Source: CAD feature listing. Evaluate the final solid. Frame: model axes, mm. A direction names the side the tool comes from. Round coordinates to 2 decimals unless told otherwise and drop trailing zeros. Order: outer loops, then holes, each group sorted by start corner. A loop starts at its lowest first (then second) coordinate and runs counter-clockwise, first axis right, second up. Notation, with made-up numbers: (-10.5, 74.25) - (26.5, 74.25) arc R21 ccw to (26.5, 97.25) - close; hole circle Ø9 at (45.5, 13.25). An arc over 180 degrees is marked (long way). Use one line per item in the form item = value. Start each with the question number.
Q1. Cut plane B-B, the plane x = -70. Return the cut outline in (y, z).
Q2. Pin query (flat end, axial travel): pin 1 Ø0.6 at (x, z) = (-142, 3) entering from -Y; pin 2 Ø1 at (x, z) = (-140, 2.5) entering from -Y; pin 3 Ø1.3 at (x, z) = (142.5, 7) entering from +Y. Return the tip coordinate at first contact, or that it passes through.
Q3. Ray query, line 1 (Y direction, x = 46, z = 8); line 2 (X direction, y = 79, z = 6.75); line 3 (Y direction, x = -70, z = 5.5). Return the intervals inside material, ascending. Write a range as [from, to].
Q4. Draft query along Y for faces 6 (the cylindrical face through (-79.74, 10.43, 4.93)), 7 (the cylindrical face through (117.09, -25.33, 5.07)), 8 (the flat face through (10, -85, 5)), 9 (the flat face through (-134, -80, 5)). Return one class per face: released by +Y, released by -Y, zero draft, split by the parting line, or undercut.
Q5. Cut plane C-C, the plane x = 34. Return the cut outline in (y, z).
Q6. Set-up query: faces 1 (the flat face through (-6, -80, 5)), 2 (the flat face through (-146, -80, 5)), 3 (the flat face through (-146, 90, 5)), 4 (the flat face through (70, -40, 5)), 5 (the flat face through (-6, 90, 5)). Return all of +Z, -Z, +X, -X, +Y, -Y with unobstructed straight access to the full face (end or side cutting, diameter ignored); none if empty.
Q7. Cut plane D-D, the plane z = 4.5. Give the number of separate pieces and of enclosed holes in the cut face, and give its area (3 significant figures).
Q8. Cut plane A-A, the plane y = -25. Return the cut outline in (x, z).
from build123d import *

# Parameters (mm, degrees)
IZIM1_W                     = 300
IZIM1_H                     = 180
IZIM1_R                     = 9.75
Y_KSEKLIK_EKSTR_ZYON1_DEPTH = 10
IZIM2_W                     = 120
IZIM2_H                     = 10
Y_KSEKLIK_EKSTR_ZYON2_DEPTH = 10
IZIM3_W                     = 20
IZIM3_H                     = 10
KES_EKSTR_ZYON1_DEPTH       = 10
IZIM4_W                     = 5.6
IZIM4_H                     = 2.7
KES_EKSTR_ZYON2_DEPTH       = 10
IZIM5_W                     = 3.2
IZIM5_H                     = 3.5
IZIM5_W_2                   = 3.168851203
IZIM5_H_2                   = 5
IZIM5_H_3                   = 5.09138305
IZIM5_W_3                   = 3.157417266
IZIM5_W_4                   = 3.164794192
IZIM5_W_5                   = 3.283155767
IZIM5_W_6                   = 3.292541888
KES_EKSTR_ZYON3_DEPTH       = 10
KES_EKSTR_ZYON4_DEPTH       = 10


with BuildPart() as part:
    # Çizim1 → Yükseklik-Ekstrüzyon1 (new body)
    with BuildSketch(Plane.XY):
        Rectangle(IZIM1_W, IZIM1_H)
        with Locations((-70, 10)):
            Circle(IZIM1_R, mode=Mode.SUBTRACT)
    extrude(amount=Y_KSEKLIK_EKSTR_ZYON1_DEPTH)

    # Çizim2 → Yükseklik-Ekstrüzyon2 (add)
    with BuildSketch(Plane(origin=(0, 90, 0), x_dir=(1, 0, 0), z_dir=(0, 1, 0))):
        with Locations((70, -5)):
            Rectangle(IZIM2_W, IZIM2_H)
        with Locations((-70, -5)):
            Rectangle(IZIM2_W, IZIM2_H)
    extrude(amount=Y_KSEKLIK_EKSTR_ZYON2_DEPTH)

    # Çizim3 → Kes-Ekstrüzyon1 (cut)
    with BuildSketch(Plane(origin=(0, -90, 0), x_dir=(-1, 0, 0), z_dir=(0, -1, 0))):
        with Locations((140, -5)):
            Rectangle(IZIM3_W, IZIM3_H)
        with Locations((-140, -5)):
            Rectangle(IZIM3_W, IZIM3_H)
        with Locations((0, -5)):
            Rectangle(IZIM3_W, IZIM3_H)
    extrude(amount=-KES_EKSTR_ZYON1_DEPTH, mode=Mode.SUBTRACT)

    # Çizim4 → Kes-Ekstrüzyon2 (cut)
    with BuildSketch(Plane.XY.offset(10)):
        with Locations((-140, 83.65)):
            Rectangle(IZIM4_W, IZIM4_H)
        with Locations((0, 83.65)):
            Rectangle(IZIM4_W, IZIM4_H)
        with Locations((140, 83.65)):
            Rectangle(IZIM4_W, IZIM4_H)
        with Locations((-140, -73.65)):
            Rectangle(IZIM4_W, IZIM4_H)
        with Locations((0, -73.65)):
            Rectangle(IZIM4_W, IZIM4_H)
        with Locations((140, -73.65)):
            Rectangle(IZIM4_W, IZIM4_H)
    extrude(amount=-KES_EKSTR_ZYON2_DEPTH, mode=Mode.SUBTRACT)

    # Çizim5 → Kes-Ekstrüzyon3 (cut)
    with BuildSketch(Plane.XY.offset(10)):
        with Locations((-140, 80.55)):
            Rectangle(IZIM5_W, IZIM5_H)
        with Locations((0, 80.55)):
            Rectangle(IZIM5_W, IZIM5_H)
        with Locations((140, 80.55)):
            Rectangle(IZIM5_W, IZIM5_H)
        with Locations((-140, -70.55)):
            Rectangle(IZIM5_W, IZIM5_H)
        with Locations((0, -70.55)):
            Rectangle(IZIM5_W, IZIM5_H)
        with Locations((-0.015574398, 87.5)):
            Rectangle(IZIM5_W_2, IZIM5_H_2)
        with Locations((140, -70.55)):
            Rectangle(IZIM5_W, IZIM5_H)
        with Locations((-140, 87.545691525)):
            Rectangle(IZIM5_W, IZIM5_H_3)
        with Locations((139.978708633, 87.5)):
            Rectangle(IZIM5_W_3, IZIM5_H_2)
        with Locations((139.982397096, -77.5)):
            Rectangle(IZIM5_W_4, IZIM5_H_2)
        with Locations((0.041577884, -77.5)):
            Rectangle(IZIM5_W_5, IZIM5_H_2)
        with Locations((-139.953729056, -77.5)):
            Rectangle(IZIM5_W_6, IZIM5_H_2)
    extrude(amount=-KES_EKSTR_ZYON3_DEPTH, mode=Mode.SUBTRACT)

    # Çizim6 → Kes-Ekstrüzyon4 (cut)
    with BuildSketch(Plane.XY.offset(10)):
        with BuildLine():
            Line((38.464975521, 60), (102.095024479, 60))
            ThreePointArc((102.095024479, 60), (117.095024479, 45), (102.095024479, 30))
            Line((102.095024479, 30), (38.464975521, 30))
            ThreePointArc((38.464975521, 30), (23.464975521, 45), (38.464975521, 60))
        make_face()
        with BuildLine():
            Line((38.464975521, -40), (102.095024479, -40))
            ThreePointArc((102.095024479, -40), (117.095024479, -25), (102.095024479, -10))
            Line((102.095024479, -10), (38.464975521, -10))
            ThreePointArc((38.464975521, -10), (23.464975521, -25), (38.464975521, -40))
        make_face()
    extrude(amount=-KES_EKSTR_ZYON4_DEPTH, mode=Mode.SUBTRACT)


solid = part.part
Completed:
q1.outline = (-90, 0) - (0.25, 0) - (0.25, 10) - (-90, 10) - close; (19.75, 0) - (100, 0) - (100, 10) - (19.75, 10) - close
q2.pin_1 = -80
q2.pin_2 = -68.8
q2.pin_3 = 90
q3.line_1 = [-90, -40], [-10, 30], [60, 100]
q3.line_2 = [-150, -141.6], [-138.4, -1.6], [1.6, 138.4], [141.6, 150]
q3.line_3 = [-90, 0.25], [19.75, 100]
q4.face_6 = undercut
q4.face_7 = undercut
q4.face_8 = zero draft
q4.face_9 = released by -Y
q5.outline = (-90, 0) - (-39.32, 0) - (-39.32, 10) - (-90, 10) - close; (-10.68, 0) - (30.68, 0) - (30.68, 10) - (-10.68, 10) - close; (59.32, 0) - (100, 0) - (100, 10) - (59.32, 10) - close
q6.face_1 = +Z, -Z, -Y
q6.face_2 = +Z, -Z, -X, -Y
q6.face_3 = +Z, -Z, -X, +Y
q6.face_4 = +Z, -Z
q6.face_5 = +Z, -Z, +Y
q7.separate_pieces = 1
q7.enclosed_holes = 3
q7.area = 50,000 mm2
q8.outline = (-150, 0) - (23.46, 0) - (23.46, 10) - (-150, 10) - close; (117.1, 0) - (150, 0) - (150, 10) - (117.1, 10) - close
